The listing builds one solid part. Answer for the finished solid, in the listing's coordinates (mm). Round coordinates to 2 decimals unless told otherwise and drop trailing zeros. Write each loop counter-clockwise with the first axis right and the second up, starting at its lowest first coordinate (ties: lowest second). Pieces come first, ordered by that corner, then holes. Notation, with made-up numbers: M 18,84 L 70,84 A18 ccw 70,108 Z; hole C 79,74 d10. An arc over 180 degrees is marked long. One line per item, written item: value. Start each with the question number.
(1) For a pull along X with two mould halves and no side action, classify faces 1 (the cylindrical face through (23.627, 3.042, 5.445)), 2 (the flat face through (-2, 3, -100)), 3 (the flat face through (145, 3, -1)) as released by +X, released by -X, zero draft, split by the parting line, or undercut.
(2) Section C-C (y = 1.6) is taken. State how many separate pieces and enclosed holes the cut face has, plus the area to 3 significant figures.
(3) Section B-B (z = 9.5) is taken. Determine the outline of the cut face in (x, y).
(4) Section A-A (x = 82.75) is taken. Determine the outline of the cut face in (y, z), plus the area to 3 significant figures.
(5) Consider probe 1 along Z at (x, y) = (46.75, 3.15); probe 2 along Z at (x, y) = (-101, 4.55); probe 3 along X at (y, z) = (2.85, 9.5). Determine where each line is inside the solid, lowest interval first.
Autodesk Inventor part; units mm, degrees
ref_plane "YZ Plane" through (0, 0, 0) normal (1, 0, 0) x (0, 1, 0)
ref_plane "XZ Plane" through (0, 0, 0) normal (0, 1, 0) x (-1, 0, 0)
ref_plane "XY Plane" through (0, 0, 0) normal (0, 0, 1) x (1, 0, 0)
sketch "Sketch1" plane through (0, 0, 0) normal (0, 1, 0) x (-1, 0, 0)
  line L0 (145, -100) -> (-145, -100)
  line L1 (-145, -100) -> (-145, 100)
  line L2 (-145, 100) -> (145, 100)
  line L3 (145, 100) -> (145, -100)
  line L4 (210, 0) -> (-210, 0)
  line L5 (0, -140) -> (0, 140)
  point P0 (0, 0)
  dimension "d30" = 290
  dimension "d31" = 200
extrude "Extrusion1" add sketch "Sketch1" along normal blind 6
sketch "Sketch2" plane through (0, 6, 0) normal (0, 1, 0) x (1, 0, 0)
  circle A0 centre (-19.75, -29.5) radius 13.5
  circle A1 centre (-82.75, -9.5) radius 13.5
  circle A2 centre (-19.75, 9.5) radius 13.5
  circle A3 centre (46.75, 29.5) radius 13.5
  circle A4 centre (82.75, 20.5) radius 13.5
  circle A5 centre (10.75, 29.5) radius 13.5
  circle A6 centre (10.75, -9.5) radius 13.5
  circle A7 centre (46.75, -9.5) radius 13.5
  circle A8 centre (82.75, -18.5) radius 13.5
  line L0 (-96.25, 43) -> (96.25, 43)
  line L1 (96.25, 43) -> (96.25, -43)
  line L2 (96.25, -43) -> (-96.25, -43)
  line L3 (-96.25, -43) -> (-96.25, 43)
  line L4 (145, 100) -> (-145, 100)
  line L5 (145, -100) -> (145, 100)
  line L6 (0, 140) -> (0, -140)
  line L7 (-210, 0) -> (210, 0)
  line L8 (-102.75, 31.5) -> (-62.75, 31.5)
  line L9 (-62.75, 31.5) -> (-62.75, -50.5)
  line L10 (-62.75, -50.5) -> (-102.75, -50.5)
  line L11 (-102.75, -50.5) -> (-102.75, 31.5)
  line L12 (-106.75, 33.8094) -> (-102.75, 36.1188)
  line L13 (-102.75, 36.1188) -> (-98.75, 33.8094)
  line L14 (-98.75, 33.8094) -> (-98.75, 29.1906)
  line L15 (-98.75, 29.1906) -> (-102.75, 26.8812)
  line L16 (-102.75, 26.8812) -> (-106.75, 29.1906)
  line L17 (-106.75, 29.1906) -> (-106.75, 33.8094)
  line L18 (-62.75, 36.1188) -> (-58.75, 33.8094)
  line L19 (-58.75, 33.8094) -> (-58.75, 29.1906)
  line L20 (-58.75, 29.1906) -> (-62.75, 26.8812)
  line L21 (-62.75, 26.8812) -> (-66.75, 29.1906)
  line L22 (-66.75, 29.1906) -> (-66.75, 33.8094)
  line L23 (-66.75, 33.8094) -> (-62.75, 36.1188)
  line L24 (-102.75, -45.8812) -> (-98.75, -48.1906)
  line L25 (-98.75, -48.1906) -> (-98.75, -52.8094)
  line L26 (-98.75, -52.8094) -> (-102.75, -55.1188)
  line L27 (-102.75, -55.1188) -> (-106.75, -52.8094)
  line L28 (-106.75, -52.8094) -> (-106.75, -48.1906)
  line L29 (-106.75, -48.1906) -> (-102.75, -45.8812)
  line L30 (-62.75, -45.8812) -> (-58.75, -48.1906)
  line L31 (-58.75, -48.1906) -> (-58.75, -52.8094)
  line L32 (-58.75, -52.8094) -> (-62.75, -55.1188)
  line L33 (-62.75, -55.1188) -> (-66.75, -52.8094)
  line L34 (-66.75, -52.8094) -> (-66.75, -48.1906)
  line L35 (-66.75, -48.1906) -> (-62.75, -45.8812)
  point P0 (-58.75, 31.5)
  point P1 (-98.75, -50.5)
  point P2 (-106.75, -50.5)
  point P3 (-66.75, -50.5)
  point P4 (-58.75, -50.5)
  dimension "d3" = 27
  dimension "d19" = 30.5
  dimension "d20" = 36
  dimension "d23" = 19
  dimension "d24" = 9
  dimension "d25" = 36
  dimension "d26" = 11
  dimension "d27" = 9
  dimension "d28" = 11
  dimension "d29" = 63
  dimension "d35" = 41
  dimension "d36" = 41
  dimension "d37" = 20
  dimension "d38" = 20
  dimension "d54" = 8
  dimension "d55" = 8
  dimension "d56" = 8
  dimension "d57" = 8
extrude "Extrusion2" cut sketch "Sketch2" against normal blind 30 contours A0 | A8 | L6 A6 L7 | A6 L6 | L30 L31 L32 L33 L34 L10 L9 | L9 L10 L34 L35 | A1 L7 | L7 A1 | L7 A2 | A2 L7 | L21 L22 L8 L9 | L9 L8 L22 L23 L18 L19 L20 | A4 | A3 | A6 L7 | L7 A7 | A7 L7 | L6 A5 | A5 L6 | L25 L26 L27 L28 L29 L11 L10 | L10 L11 L24 L25 | L14 L15 L11 L8 | L8 L11 L16 L17 L12 L13 L14 picked at (6.7806, -6.3333)
equation "\"d30\" = BoxLength"
equation "\"d31\" = BoxWidth"
equation "\"d3\" = JS_Hole_dia"
equation "\"d36\" = 0.5 * JS_SH_L"
equation "\"d37\" = 0.5 * JS_SH_W"
equation "\"d38\" = 0.5 * JS_SH_W"
equation "\"BoxLength\" = 290"
equation "\"BoxWidth\" = 200"
equation "\"JS_SH_L\" = 82"
equation "\"JS_SH_dia\" = 5"
equation "\"SheetThickness\" = 6"
equation "\"CornerOffset\" = 5"
equation "\"NutS\" = 5.7"
equation "\"NutThreadD2\" = 4.17"
equation "\"SideNutWidth\" = 2.5"
equation "\"JS_Hole_dia\" = 27"
equation "\"JS_SH_hex_width\" = 8"
properties part number "sega_straight_b1_v2"
Recorded:
1. face 1: undercut
1. face 2: zero draft
1. face 3: released by +X
2. separate pieces: 1
2. enclosed holes: 13
2. area: 52,600 mm2
3. outline: M -145,0 L -96.25,0 L -96.25,6 L -145,6 Z; M -69.25,0 L -2.75,0 L -2.75,6 L -69.25,6 Z; M 24.25,0 L 33.25,0 L 33.25,6 L 24.25,6 Z; M 60.25,0 L 72.69,0 L 72.69,6 L 60.25,6 Z; M 92.81,0 L 145,0 L 145,6 L 92.81,6 Z
4. outline: M 0,-100 L 6,-100 L 6,-34 L 0,-34 Z; M 0,-7 L 6,-7 L 6,5 L 0,5 Z; M 0,32 L 6,32 L 6,100 L 0,100 Z
4. area: 876 mm2
5. probe 1: z = -100 to -43, -16 to -4, 23 to 100
5. probe 2: z = -100 to -35.11, -27.89 to 46.89, 54.11 to 100
5. probe 3: x = -145 to -96.25, -69.25 to -2.75, 24.25 to 33.25, 60.25 to 72.69, 92.81 to 145
